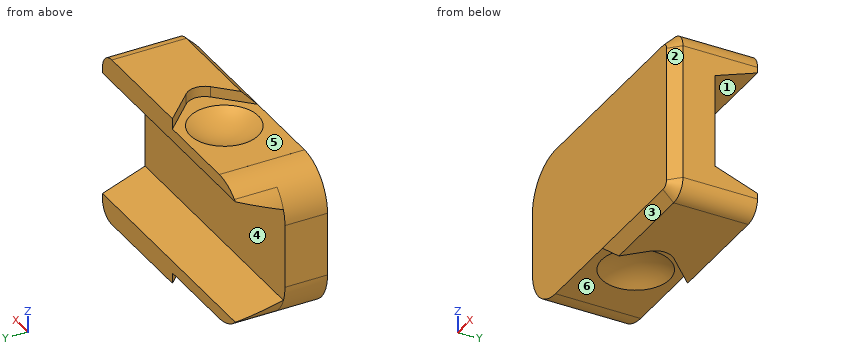
from build123d import *

# Parameters (mm, degrees)
BOSS_EXTRUDE1_DEPTH = 12.7
SKETCH2_W           = 19.05
SKETCH2_H           = 6.35
CUT_EXTRUDE1_DEPTH  = 43.121134838
CHAMFER1_START      = -18.648360593
CHAMFER1_DEPTH      = 37.698360593
CHAMFER1_START_2    = 6.35
CHAMFER1_2_DEPTH    = 7.65
CUT_EXTRUDE3_DEPTH  = 1.5875
CHAMFER3_SIZE       = 1.5875


with BuildPart() as part:
    # Sketch1 → Boss-Extrude1 (new body)
    with BuildSketch(Plane(origin=(0, 0, 0), x_dir=(1, 0, 0), z_dir=(0, 1, 0))):
        with BuildLine():
            Line((-11.189157294, -12.7), (16.51, -12.7))
            ThreePointArc((16.51, -12.7), (18.306051224, -11.956051224), (19.05, -10.16))
            Line((19.05, -10.16), (19.05, 10.16))
            ThreePointArc((19.05, 10.16), (18.306051224, 11.956051224), (16.51, 12.7))
            Line((16.51, 12.7), (-11.189157294, 12.7))
            Line((-11.189157294, 12.7), (-12.777125687, 11.112031607))
            ThreePointArc((-12.777125687, 11.112031607), (-17.21731381, 9.225276708), (-19.05, 4.7625))
            Line((-19.05, 4.7625), (-19.05, -4.7625))
            ThreePointArc((-19.05, -4.7625), (-17.21731381, -9.225276708), (-12.777125687, -11.112031607))
            Line((-12.777125687, -11.112031607), (-11.189157294, -12.7))
        make_face()
    extrude(amount=BOSS_EXTRUDE1_DEPTH)

    # Sketch2 → Cut-Extrude1 (cut, through all)
    with BuildSketch(Plane.ZY.offset(19.05)):
        with Locations((0, 9.525)):
            Rectangle(SKETCH2_W, SKETCH2_H)
    extrude(amount=-CUT_EXTRUDE1_DEPTH, mode=Mode.SUBTRACT)

    # Chamfer1: read off the stored shape, not the designer's step
    # Chamfer1 outline → Chamfer1 (add)
    with BuildSketch(Plane.YZ.offset(CHAMFER1_START)):
        Polygon((6.35, 9.525), (6.35, 6.985), (12.7, 9.296210988), (12.7, 9.525), align=None)
        Polygon((12.7, -9.296210988), (6.35, -6.985), (6.35, -9.525), (12.7, -9.525), align=None)
    extrude(amount=CHAMFER1_DEPTH)

    # Chamfer1 2 outline → Chamfer1 2 (cut)
    with BuildSketch(Plane(origin=(0, 0, 0), x_dir=(1, 0, 0), z_dir=(0, 1, 0)).offset(CHAMFER1_START_2)):
        with BuildLine():
            Line((-18.648360593, -9.525), (-16.900130206, -9.525))
            ThreePointArc((-16.900130206, -9.525), (-17.930761549, -8.362726885), (-18.648360594, -6.985))
            Line((-18.648360594, -6.985), (-18.648360593, -9.525))
        make_face()
        with BuildLine():
            Line((-18.648360593, 9.525), (-18.648360594, 6.985))
            ThreePointArc((-18.648360594, 6.985), (-17.930761549, 8.362726885), (-16.900130206, 9.525))
            Line((-16.900130206, 9.525), (-18.648360593, 9.525))
        make_face()
    extrude(amount=CHAMFER1_2_DEPTH, mode=Mode.SUBTRACT)

    # Sketch4 → Cut-Extrude3 (cut)
    with BuildSketch(Plane.XY.offset(12.7)):
        with BuildLine():
            Line((-19.05, 0), (0, 0))
            Line((0, 0), (4.553948776, 4.553948776))
            ThreePointArc((4.553948776, 4.553948776), (5.297897552, 6.35), (4.553948776, 8.146051224))
            Line((4.553948776, 8.146051224), (0, 12.7))
            Line((0, 12.7), (-19.05, 12.7))
            Line((-19.05, 12.7), (-19.05, 0))
        make_face()
    cut_extrude3 = extrude(amount=-CUT_EXTRUDE3_DEPTH, mode=Mode.SUBTRACT)

    # Sketch6 → Cut-Revolve1 (revolve, cut)
    with BuildSketch(Plane.ZY.offset(2.54)):
        with BuildLine():
            Line((11.1125, 6.35), (11.1125, 11.43))
            ThreePointArc((11.1125, 11.43), (9.931118256, 9.01113492), (9.525, 6.35))
            Line((9.525, 6.35), (11.1125, 6.35))
        make_face()
    cut_revolve1 = revolve(axis=Axis((-2.54, 6.35, 0), (0, 0, 1)), mode=Mode.SUBTRACT)

    # Mirror1: Cut-Extrude3, Cut-Revolve1 across plane
    add(cut_extrude3.mirror(Plane(origin=(0, 0, 0), x_dir=(1, 0, 0), z_dir=(0, 0, -1))), mode=Mode.SUBTRACT)
    add(cut_revolve1.mirror(Plane(origin=(0, 0, 0), x_dir=(1, 0, 0), z_dir=(0, 0, -1))), mode=Mode.SUBTRACT)

    # Chamfer3
    chamfer3_edges = [part.edges().sort_by_distance(p)[0] for p in [
        (8.255, 0, 12.7),
        (18.306051224, 0, 11.956051224),
        (19.05, 0, 0),
        (18.306051224, 0, -11.956051224),
        (8.255, 0, -12.7),
    ]]
    chamfer(chamfer3_edges, length=CHAMFER3_SIZE)


solid = part.part
Geometry check sheet. Reference: the model listing, model coordinates, mm. Face numbers are marked on the shaded views. A direction names the side the tool comes from. Give positions to 0.01 mm unless a question says otherwise; leave off trailing zeros. Loops run counter-clockwise (first coordinate to the right, second up) from the corner with the lowest first, then second, coordinate; pieces in that order, holes last. Notation, with made-up numbers: M -16.5,-18 L 19.5,-18 A14 ccw 19.5,5 Z; hole C 54.5,66 d9. An arc over 180 degrees is marked long. Answer as a JSON object with one key per item and string values. Group by question number.
Item 1: Sectioned sample at B-B on z = 2.5. Record the boundary of the cut face in (x, y), plus the area to 3 significant figures.
Item 2: Gauge pin test, flat ends, axial feed: pin 1 (3 mm diameter, centred on x = 2.5, z = 3.5, fed in from +Y); pin 2 (3 mm diameter, centred on x = -11, y = 8.5, fed in from -Z). Record the tip position at first contact, or that the pin passes through.
Item 3: Access from +Z, -Z, +X, -X, +Y, -Y to the whole of each face (thin tool, end or side, straight path). Record for the marked faces 4, 5 and 6.
Item 4: Mould release check, pull along Z, two halves, no side actions. Record for the marked faces 1, 2 and 3: pulls with the +Z half, pulls with the -Z half, needs draft (parallel to the pull), parting line crosses it, or undercut.
Item 5: Material ranges on L1, parallel to Y at x = -14, z = 1.5; L2, parallel to Z at x = -15, y = 11.5; L3, parallel to Z at x = -14, y = 11.5, recorded low to high.
Findings below:
{
 "1": {"outline": "M -19.05,0 L 17.46,0 L 19.05,1.59 L 19.05,6.35 L -19.05,6.35 Z", "area": "241 mm2"},
 "2": {"pin 1": "y = 6.35", "pin 2": "z = -11.11"},
 "3": {"face 4": "+X, -X, +Y", "face 5": "+Z, -X", "face 6": "-Z, -X"},
 "4": {"face 1": "undercut", "face 2": "needs draft", "face 3": "pulls with the -Z half"},
 "5": {"L1": "0 to 6.35", "L2": "-10.68 to -8.86, 8.86 to 10.68", "L3": "-10.98 to -8.86, 8.86 to 10.98"}
}
